```python
from build123d import *

# Parameters (mm, degrees)
ESQUISSE1_R        = 3
BOSS_EXTRU_1_DEPTH = 20
D_ME1_FACE_RADIUS  = 3
D_ME1_HEIGHT       = 1
D_ME2_FACE_RADIUS  = 3
D_ME2_HEIGHT       = 1


with BuildPart() as part:
    # Esquisse1 → Boss.-Extru.1 (new body)
    with BuildSketch(Plane(origin=(0, 0, 0), x_dir=(1, 0, 0), z_dir=(0, 1, 0))):
        with Locations(Location((0, 0, 0), (0, 0, 270))):
            Circle(ESQUISSE1_R)
    extrude(amount=BOSS_EXTRU_1_DEPTH)

    # D_me1: an elliptical dome of height H over a round flat face of radius A is half a spheroid: the quarter ellipse of half axes A and H revolved about the face's axis
    with BuildSketch(Plane((0, 20, 0), x_dir=(0, 0, -1), z_dir=(1, 0, 0)), mode=Mode.PRIVATE) as d_me1_quarter:
        Ellipse(D_ME1_FACE_RADIUS, D_ME1_HEIGHT)
        Rectangle(D_ME1_FACE_RADIUS, D_ME1_HEIGHT, align=(Align.MIN, Align.MIN), mode=Mode.INTERSECT)
    revolve(d_me1_quarter.sketch, axis=Axis((0, 20, 0), (0, 1, 0)))

    # D_me2: an elliptical dome of height H over a round flat face of radius A is half a spheroid: the quarter ellipse of half axes A and H revolved about the face's axis
    with BuildSketch(Plane((0, 0, 0), x_dir=(0, 0, 1), z_dir=(1, 0, 0)), mode=Mode.PRIVATE) as d_me2_quarter:
        Ellipse(D_ME2_FACE_RADIUS, D_ME2_HEIGHT)
        Rectangle(D_ME2_FACE_RADIUS, D_ME2_HEIGHT, align=(Align.MIN, Align.MIN), mode=Mode.INTERSECT)
    revolve(d_me2_quarter.sketch, axis=Axis((0, 0, 0), (0, -1, 0)))


solid = part.part
```
Work out the finished part from the listing and answer in its coordinate system (mm). Coordinates: 2 decimals unless noted, no trailing zeros. Order: outer loops, then holes, each group sorted by start corner. A loop starts at its lowest first (then second) coordinate and runs counter-clockwise, first axis right, second up. Notation, with made-up numbers: (51, 79.5) - (91, 79.5) arc R24 cw to (91, 104.5) - close; hole circle Ø8 at (5.25, -10). An arc over 180 degrees is marked (long way). Answer as a JSON object with one key per item and string values.
1. Consider line 1 (Y direction, x = 0, z = -1.25); line 2 (Z direction, x = 2.75, y = 1.25); line 3 (X direction, y = 14.25, z = -0.5). Determine where each line is inside the solid, lowest interval first.
Output values:
{"line 1": "y = -0.91 to 20.91", "line 2": "z = -1.2 to 1.2", "line 3": "x = -2.96 to 2.96"}
2. Find section A-A on y = 9. Determine the outline of the cut face in (x, z).
Output values:
{"outline": "circle Ø6 at (0, 0)"}
3. Each of these flat-tipped pins is pushed along its axis until it touches: P1, Ø2, axis at y = 12.5, z = 2.5, coming from the -X side; P2, Ø1.5, axis at x = -1.5, y = 14, coming from the -Z side; P3, Ø1, axis at y = 6, z = 1.5, coming from the -X side. Where does it stop, or does it pass through?
Output values:
{"P1": "stops at x = -2.6", "P2": "stops at z = -2.9", "P3": "stops at x = -2.83"}
